from build123d import *

# Parameters (mm, degrees)
SKETCH1_W           = 1.6
SKETCH1_H           = 20
BOSS_EXTRUDE1_DEPTH = 45
SKETCH2_W           = 10
SKETCH2_H           = 2.5
BOSS_EXTRUDE2_DEPTH = 2.5
SKETCH3_W           = 0.8
SKETCH3_H           = 0.8
BOSS_EXTRUDE3_DEPTH = 9
SKETCH4_R           = 8
BOSS_EXTRUDE4_DEPTH = 12
SKETCH5_R           = 7
CUT_EXTRUDE1_DEPTH  = 1


with BuildPart() as part:
    # Sketch1 → Boss-Extrude1 (new body)
    with BuildSketch(Plane.XY):
        Rectangle(SKETCH1_W, SKETCH1_H)
    extrude(amount=BOSS_EXTRUDE1_DEPTH)

    # Sketch2 → Boss-Extrude2 (add)
    with BuildSketch(Plane(origin=(0.8, 0, 0), x_dir=(0, 0, -1), z_dir=(1, 0, 0))):
        with Locations((-22.5, -8.25)):
            Rectangle(SKETCH2_W, SKETCH2_H)
    extrude(amount=BOSS_EXTRUDE2_DEPTH)

    # Sketch3 → Boss-Extrude3 (add)
    with BuildSketch(Plane(origin=(3.3, -6.2, 0), x_dir=(0, -1, 0), z_dir=(-1, 0, 0))):
        with Locations((2.000946282, 26.25)):
            Rectangle(SKETCH3_W, SKETCH3_H)
        with Locations((2.000946282, 23.75)):
            Rectangle(SKETCH3_W, SKETCH3_H)
        with Locations((2.000946282, 21.25)):
            Rectangle(SKETCH3_W, SKETCH3_H)
        with Locations((2.000946282, 18.75)):
            Rectangle(SKETCH3_W, SKETCH3_H)
    extrude(amount=-BOSS_EXTRUDE3_DEPTH)

    # Sketch4 → Boss-Extrude4 (add)
    with BuildSketch(Plane.ZY.offset(0.8)):
        with Locations(Location((9.5, 0, 0), (0, 0, 180))):
            Circle(SKETCH4_R)
        with Locations(Location((35.5, 0, 0), (0, 0, 180))):
            Circle(SKETCH4_R)
    extrude(amount=BOSS_EXTRUDE4_DEPTH)

    # Sketch5 → Cut-Extrude1 (cut)
    with BuildSketch(Plane.ZY.offset(12.8)):
        with Locations((35.5, 0)):
            Circle(SKETCH5_R)
        with Locations((9.5, 0)):
            Circle(SKETCH5_R)
    extrude(amount=-CUT_EXTRUDE1_DEPTH, mode=Mode.SUBTRACT)


solid = part.part
The listing builds one solid part. Answer for the finished solid, in the listing's coordinates (mm). A direction names the side the tool comes from. Give positions to 0.01 mm unless a question says otherwise; leave off trailing zeros. Order: outer loops, then holes, each group sorted by start corner. A loop starts at its lowest first (then second) coordinate and runs counter-clockwise, first axis right, second up. Notation, with made-up numbers: (-20.75, -15) -> (31.25, -15) arc R23 cw to (31.25, 6) -> close; hole circle Ø1 at (11.5, 8.5). An arc over 180 degrees is marked (long way). Put each result on its own line as item: value.
Item 1: A cutting plane is placed at C-C on z = 9.5. Give the vertices of the cut face in (x, y), plus the area to 3 significant figures.
Established:
outline: (-12.8, -8) -> (-0.8, -8) -> (-0.8, -10) -> (0.8, -10) -> (0.8, 10) -> (-0.8, 10) -> (-0.8, 8) -> (-12.8, 8) -> (-12.8, 7) -> (-11.8, 7) -> (-11.8, -7) -> (-12.8, -7) -> close
area: 210 mm^2
Item 2: Given P1, Ø3, axis at y = 2, z = 36.5, coming from the +X side; P2, Ø0.8, axis at x = 2, z = 23.5, coming from the +Y side; P3, Ø0.9, axis at x = 7.5, y = -8, coming from the +Z side; P4, Ø12, axis at x = -1, z = 34.5, coming from the -Y side, each flat-ended and moving along its own axis, determine where each tip first touches the part or whether it passes through.
Established:
P1: stops at x = 0.8
P2: stops at y = -7
P3: stops at z = 26.65
P4: stops at y = -10
Item 3: A cutting plane is placed at D-D on x = -5.5. Give the vertices of the cut face in (y, z), plus the area to 3 significant figures.
Established:
outline: circle Ø16 at (0, 9.5); circle Ø16 at (0, 35.5)
area: 402 mm^2
Item 4: A cutting plane is placed at A-A on y = 0. Give the vertices of the cut face in (x, z).
Established:
outline: (-12.8, 1.5) -> (-0.8, 1.5) -> (-0.8, 0) -> (0.8, 0) -> (0.8, 45) -> (-0.8, 45) -> (-0.8, 43.5) -> (-12.8, 43.5) -> (-12.8, 42.5) -> (-11.8, 42.5) -> (-11.8, 28.5) -> (-12.8, 28.5) -> (-12.8, 27.5) -> (-0.8, 27.5) -> (-0.8, 17.5) -> (-12.8, 17.5) -> (-12.8, 16.5) -> (-11.8, 16.5) -> (-11.8, 2.5) -> (-12.8, 2.5) -> close
Item 5: Straight lines are drawn through the part: line 1 (Y direction, x = -12.1, z = 35.5); line 2 (X direction, y = -4.5, z = 37); line 3 (X direction, y = 9, z = 11). For each, find the intervals that lie inside material, in ascending order.
Established:
line 1: y = -8 to -7, 7 to 8
line 2: x = -11.8 to 0.8
line 3: x = -0.8 to 0.8
Item 6: For a pull along Z with two mould halves and no side action, classify faces 6 (the face through (2, -8, 27.5)), 7 (the face through (-0.8, 0, 22)), 8 (the face through (0, 0, 0)) as released by +Z, released by -Z, zero draft, split by the parting line, or undercut.
Established:
face 6: released by +Z
face 7: undercut
face 8: released by -Z
Item 7: For faces 1 (the face through (2, -8, 17.5)), 2 (the face through (2, -9.5, 23)), 3 (the face through (-12.307, 2.103, 42.177)), 4 (the face through (2, -7, 23)), 5 (the face through (0, -10, 22)), determine the directions among +Z, -Z, +X, -X, +Y, -Y from which every point of the face is accessible in a straight line to the end or side of a thin tool.
Established:
face 1: -Z, +X, +Y, -Y
face 2: +Z, -Z, +X, -Y
face 3: -X
face 4: +Z, -Z, +X, +Y
face 5: +Z, -Z, +X, -X, -Y
Item 8: A cutting plane is placed at B-B on x = 8.5. Give the vertices of the cut face in (y, z).
Established:
outline: (-8.6, 18.35) -> (-7.8, 18.35) -> (-7.8, 19.15) -> (-8.6, 19.15) -> close; (-8.6, 20.85) -> (-7.8, 20.85) -> (-7.8, 21.65) -> (-8.6, 21.65) -> close; (-8.6, 23.35) -> (-7.8, 23.35) -> (-7.8, 24.15) -> (-8.6, 24.15) -> close; (-8.6, 25.85) -> (-7.8, 25.85) -> (-7.8, 26.65) -> (-8.6, 26.65) -> close
